Design review of the part built by this model. Coordinates are the model's own, in mm. A direction names the side the tool comes from. Coordinates: 2 decimals unless noted, no trailing zeros. Write each loop counter-clockwise with the first axis right and the second up, starting at its lowest first coordinate (ties: lowest second). Pieces come first, ordered by that corner, then holes.
Q1. Machinability: for faces 1 (the face through (45, -20, 10)), 2 (the face through (-1, 47, 15)), 3 (the face through (-1, -65, 22)), 4 (the face through (27.5, 77, 11)), 5 (the face through (40.25, -4, 4)), which of the approach directions +Z, -Z, +X, -X, +Y, -Y give a long, thin tool a straight path to every point of the face, cutting with its end or side? Answer none if there is none.
Q2. Clearance check with flat-ended pins moving along their axes: pin 1 Ø3 at (x, y) = (25.5, 5.5) entering from -Z; pin 2 Ø4 at (x, z) = (-9.5, 13) entering from +Y. State where each tip first meets the part, or that it passes through.
Q3. Add section D-D, the plane y = 48. Give the boundary of the cut face in (x, z), plus the area to 3 significant figures.
Q4. Add section C-C, the plane y = -18.5. Give the boundary of the cut face in (x, z).
Q5. Add section A-A, the plane z = 4. Give the boundary of the cut face in (x, y).
Q6. Add section B-B, the plane y = 71.5. Give the boundary of the cut face in (x, z).
Q7. To check wall thickness, follow probe 1 along X at (y, z) = (-42.5, 8.75); probe 2 along X at (y, z) = (-12.5, 5.5); probe 3 along Z at (x, y) = (-34, 40). State the ranges of each line that lie inside material, in increasing order.
from build123d import *

# Parameters (mm, degrees)
SKETCH_1_W          = 90
SKETCH_1_H          = 170
EXTRUDE_1_DEPTH     = 25
SKETCH_2_W          = 90
SKETCH_2_H          = 70.292308138
CUT_EXTRUDE_1_DEPTH = 10
FILLET_1_R          = 10
FILLET_2_R          = 10
SKETCH_3_W          = 80.5
SKETCH_3_H          = 165.25
CUT_EXTRUDE_2_DEPTH = 10
SKETCH_5_W          = 0.6
SKETCH_5_H          = 165.25
EXTRUDE_2_DEPTH     = 0.9
SKETCH_6_W          = 0.6
SKETCH_6_H          = 165.25
EXTRUDE_3_DEPTH     = 0.9
SKETCH_9_W          = 90
SKETCH_9_H          = 10
CUT_EXTRUDE_5_DEPTH = 3
FILLET_8_R          = 1
FILLET_9_R          = 1
SKETCH_10_W         = 55
SKETCH_10_H         = 40
CUT_EXTRUDE_6_DEPTH = 20


with BuildPart() as part:
    # 草图1 → 凸台-拉伸1 (new body)
    with BuildSketch(Plane.XY):
        Rectangle(SKETCH_1_W, SKETCH_1_H)
    extrude(amount=EXTRUDE_1_DEPTH)

    # 草图2 → 切除-拉伸1 (cut)
    with BuildSketch(Plane.XY.offset(25)):
        with Locations((0, 49.853845931)):
            Rectangle(SKETCH_2_W, SKETCH_2_H)
    extrude(amount=-CUT_EXTRUDE_1_DEPTH, mode=Mode.SUBTRACT)

    # 圆角1
    fillet_1_edges = [part.edges().sort_by_distance(p)[0] for p in [
        (0, 14.707691862, 25),
    ]]
    fillet(fillet_1_edges, radius=FILLET_1_R - 0.0001)  # a hair under: the kernel refuses the full size

    # 圆角2
    fillet_2_edges = [part.edges().sort_by_distance(p)[0] for p in [
        (0, 14.707691862, 15),
    ]]
    fillet(fillet_2_edges, radius=FILLET_2_R)

    # 草图3 → 切除-拉伸2 (cut)
    with BuildSketch(Plane(origin=(0, 0, 0), x_dir=(-1, 0, 0), z_dir=(0, 0, -1))):
        with Locations((0, -2.375)):
            Rectangle(SKETCH_3_W, SKETCH_3_H)
    extrude(amount=-CUT_EXTRUDE_2_DEPTH, mode=Mode.SUBTRACT)

    # 草图5 → 凸台-拉伸2 (add)
    with BuildSketch(Plane.ZY.offset(-40.25)):
        with Locations((8.5, -2.375)):
            Rectangle(SKETCH_5_W, SKETCH_5_H)
    extrude(amount=EXTRUDE_2_DEPTH)

    # 草图6 → 凸台-拉伸3 (add)
    with BuildSketch(Plane(origin=(-40.25, 0, 0), x_dir=(0, 0, -1), z_dir=(1, 0, 0))):
        with Locations((-9.1, -2.375)):
            Rectangle(SKETCH_6_W, SKETCH_6_H)
    extrude(amount=EXTRUDE_3_DEPTH)

    # 草图9 → 切除-拉伸5 (cut)
    with BuildSketch(Plane.XY.offset(25)):
        with Locations((0, -65.064201391)):
            Rectangle(SKETCH_9_W, SKETCH_9_H)
    extrude(amount=-CUT_EXTRUDE_5_DEPTH, mode=Mode.SUBTRACT)

    # 圆角8
    fillet_8_edges = [part.edges().sort_by_distance(p)[0] for p in [
        (0, -60.064201391, 22),
        (0, -60.064201391, 25),
    ]]
    fillet(fillet_8_edges, radius=FILLET_8_R)

    # 圆角9
    fillet_9_edges = [part.edges().sort_by_distance(p)[0] for p in [
        (0, -70.064201391, 22),
        (0, -70.064201391, 25),
    ]]
    fillet(fillet_9_edges, radius=FILLET_9_R)

    # 草图10 → 切除-拉伸6 (cut)
    with BuildSketch(Plane.XY.offset(15)):
        with Locations((0, 85)):
            Rectangle(SKETCH_10_W, SKETCH_10_H)
    extrude(amount=-CUT_EXTRUDE_6_DEPTH, mode=Mode.SUBTRACT)


solid = part.part
Here are the results:
1. face 1: +Z, -Z, +X, +Y, -Y
1. face 2: +Z, +X, -X, +Y
1. face 3: +Z, +X, -X
1. face 4: +Z, -Z, +Y
1. face 5: -Z, -Y
2. pin 1: stops at z = 10
2. pin 2: stops at y = 65
3. outline: (-45, 0) - (-40.25, 0) - (-40.25, 8.8) - (-39.35, 8.8) - (-39.35, 9.4) - (-40.25, 9.4) - (-40.25, 10) - (40.25, 10) - (40.25, 8.8) - (39.35, 8.8) - (39.35, 8.2) - (40.25, 8.2) - (40.25, 0) - (45, 0) - (45, 15) - (-45, 15) - close
3. area: 546 mm2
4. outline: (-45, 0) - (-40.25, 0) - (-40.25, 8.8) - (-39.35, 8.8) - (-39.35, 9.4) - (-40.25, 9.4) - (-40.25, 10) - (40.25, 10) - (40.25, 8.8) - (39.35, 8.8) - (39.35, 8.2) - (40.25, 8.2) - (40.25, 0) - (45, 0) - (45, 25) - (-45, 25) - close
5. outline: (-45, -85) - (-40.25, -85) - (-40.25, 80.25) - (-27.5, 80.25) - (-27.5, 85) - (-45, 85) - close; (27.5, 80.25) - (40.25, 80.25) - (40.25, -85) - (45, -85) - (45, 85) - (27.5, 85) - close
6. outline: (-45, 0) - (-40.25, 0) - (-40.25, 8.8) - (-39.35, 8.8) - (-39.35, 9.4) - (-40.25, 9.4) - (-40.25, 10) - (-27.5, 10) - (-27.5, 15) - (-45, 15) - close; (27.5, 10) - (40.25, 10) - (40.25, 8.8) - (39.35, 8.8) - (39.35, 8.2) - (40.25, 8.2) - (40.25, 0) - (45, 0) - (45, 15) - (27.5, 15) - close
7. probe 1: x = -45 to -40.25, 39.35 to 45
7. probe 2: x = -45 to -40.25, 40.25 to 45
7. probe 3: z = 10 to 15
